Here's how the part is built. I have some questions about the finished solid (model axes, mm). Face numbers are marked on the shaded views. A direction names the side the tool comes from. Round coordinates to 2 decimals unless told otherwise and drop trailing zeros. Loops run counter-clockwise (first coordinate to the right, second up) from the corner with the lowest first, then second, coordinate; pieces in that order, holes last. Notation, with made-up numbers: M 48,13 L 69,13 A21 cw 69,48 Z; hole C 62.25,78.5 d6. An arc over 180 degrees is marked long. Answer as a JSON object with one key per item and string values.
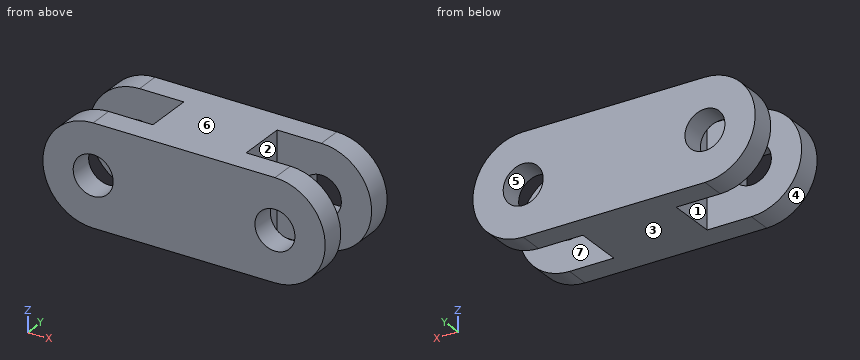
from build123d import *

# Parameters (mm, degrees)
SKETCH1_R           = 1.65
BOSS_EXTRUDE1_DEPTH = 2
SKETCH2_W           = 7.7
SKETCH2_H           = 8.3
BOSS_EXTRUDE2_DEPTH = 1


with BuildPart() as part:
    # Sketch1 → Boss-Extrude1 (new body)
    with BuildSketch(Plane(origin=(0, 0, 0), x_dir=(1, 0, 0), z_dir=(0, 1, 0))):
        with BuildLine():
            Line((-7.5, 4.15), (7.5, 4.15))
            ThreePointArc((7.5, 4.15), (11.65, 0), (7.5, -4.15))
            Line((7.5, -4.15), (-7.5, -4.15))
            ThreePointArc((-7.5, -4.15), (-11.65, 0), (-7.5, 4.15))
        make_face()
        with Locations(Location((-7.5, 0, 0), (0, 0, 270))):
            Circle(SKETCH1_R, mode=Mode.SUBTRACT)
        with Locations(Location((7.5, 0, 0), (0, 0, 270))):
            Circle(SKETCH1_R, mode=Mode.SUBTRACT)
    extrude(amount=BOSS_EXTRUDE1_DEPTH)

    # Sketch2 → Boss-Extrude2 (add)
    with BuildSketch(Plane(origin=(0, 2, 0), x_dir=(1, 0, 0), z_dir=(0, 1, 0))):
        Rectangle(SKETCH2_W, SKETCH2_H)
    boss_extrude2 = extrude(amount=BOSS_EXTRUDE2_DEPTH)

    # Mirror1: Boss-Extrude2 across plane
    add(boss_extrude2.mirror(Plane.ZX.offset(3)))

    # Mirror4: part across plane


with BuildPart() as part_1:
    add(part.part)
    add(part.part.mirror(Plane(origin=(0, 4, 0), x_dir=(0, 0, 1), z_dir=(0, -1, 0))))


solid = part_1.part
Item 1: For P1, Ø1.5, axis at y = 4.5, z = 2.5, coming from the +X side; P2, Ø1.2, axis at y = 5, z = 1, coming from the -X side, each with a flat end and sliding along its axis, tell me the tip position at first contact or that it passes through.
Solution:
{"P1": "stops at x = 3.85", "P2": "stops at x = -3.85"}
Item 2: I want a section at A-A on z = 0. List the corners of the cut face in (x, y) for me.
Solution:
{"outline": "M -11.65,0 L -9.15,0 L -9.15,2 L -11.65,2 Z; M -11.65,6 L -9.15,6 L -9.15,8 L -11.65,8 Z; M -5.85,0 L 5.85,0 L 5.85,2 L 3.85,2 L 3.85,6 L 5.85,6 L 5.85,8 L -5.85,8 L -5.85,6 L -3.85,6 L -3.85,2 L -5.85,2 Z; M 9.15,0 L 11.65,0 L 11.65,2 L 9.15,2 Z; M 9.15,6 L 11.65,6 L 11.65,8 L 9.15,8 Z"}
Item 3: I want a section at B-B on x = 5. List the corners of the cut face in (y, z) for me, plus the area to 3 significant figures.
Solution:
{"outline": "M 0,-4.15 L 2,-4.15 L 2,4.15 L 0,4.15 Z; M 6,-4.15 L 8,-4.15 L 8,4.15 L 6,4.15 Z", "area": "33.2 mm2"}
Item 4: If I drill on L1, parallel to X at y = 0.7, z = 0; L2, parallel to Y at x = -7.5, z = 3; L3, parallel to X at y = 6.5, z = 1, over which ranges is the centre line in solid material (lowest first)? Write a range as from..to.
Solution:
{"L1": "x = -11.65..-9.15, -5.85..5.85, 9.15..11.65", "L2": "y = 0..2, 6..8", "L3": "x = -11.53..-8.81, -6.19..6.19, 8.81..11.53"}
Item 5: For the marked faces 1, 2 and 3, which set-ups out of +Z, -Z, +X, -X, +Y, -Y let a thin tool reach every point of the face, with its end or its side?
Solution:
{"face 1": "+Z, -Z, -X", "face 2": "+Z, -Z, +X", "face 3": "-Z, +X, -X, +Y, -Y"}
Item 6: I want a section at C-C on y = 7.75. List the corners of the cut face in (x, z) for me.
Solution:
{"outline": "M -7.5,-4.15 L 7.5,-4.15 A4.15 ccw 7.5,4.15 L -7.5,4.15 A4.15 ccw Z; hole C -7.5,0 d3.3; hole C 7.5,0 d3.3"}
Item 7: I want a section at D-D on x = 8.25. List the corners of the cut face in (y, z) for me, plus the area to 3 significant figures.
Solution:
{"outline": "M 0,-4.08 L 2,-4.08 L 2,-1.47 L 0,-1.47 Z; M 0,1.47 L 2,1.47 L 2,4.08 L 0,4.08 Z; M 6,-4.08 L 8,-4.08 L 8,-1.47 L 6,-1.47 Z; M 6,1.47 L 8,1.47 L 8,4.08 L 6,4.08 Z", "area": "20.9 mm2"}
Item 8: We'd pull the mould along Z, two halves only. Please class the marked faces 4, 5, 6 and 7: +Z half, -Z half, draft (parallel to the pull), parting line (faces both ways), or undercut.
Solution:
{"face 4": "parting line", "face 5": "undercut", "face 6": "+Z half", "face 7": "draft"}
